from build123d import *

# Parameters (mm, degrees)
SKETCH1_R           = 10
SKETCH1_R_2         = 3.499999985
SKETCH1_R_3         = 3.5
BOSS_EXTRUDE1_DEPTH = 3.175
CUT_EXTRUDE1_DEPTH  = 3.175


with BuildPart() as part:
    # Sketch1 → Boss-Extrude1 (new body)
    # profile 1 of 4: a face of its own
    with BuildSketch(Plane(origin=(0, 79.166310833, -2.766864901), x_dir=(0, -0.03492870325036397, -0.9993898066766781), z_dir=(0, -0.9993898066766781, 0.03492870325036397))):
        with BuildLine():
            ThreePointArc((-118.870418158, 10), (-111.799350346, 7.071067812), (-108.870418158, 0))
            ThreePointArc((-108.870418158, 0), (-111.799350346, -7.071067812), (-118.870418158, -10))
            ThreePointArc((-118.870418158, -10), (4.966133868, -24.680117915), (121.938173717, -67.906722838))
            ThreePointArc((121.938173717, -67.906722838), (119.088657305, -52.269505992), (134.924502551, -53.636363636))
            ThreePointArc((134.924502551, -53.636363636), (119.323202161, 0), (134.924502551, 53.636363636))
            ThreePointArc((134.924502551, 53.636363636), (119.088657305, 52.269505992), (121.938173717, 67.906722838))
            ThreePointArc((121.938173717, 67.906722838), (4.966133868, 24.680117915), (-118.870418158, 10))
        make_face()
    # profile 2 of 4: a face of its own
    with BuildSketch(Plane(origin=(0, 79.166310833, -2.766864901), x_dir=(0, -0.03492870325036397, -0.9993898066766781), z_dir=(0, -0.9993898066766781, 0.03492870325036397))):
        with Locations((-118.870418158, 0)):
            Circle(SKETCH1_R)
        with Locations((-118.870418158, 0)):
            Circle(SKETCH1_R_2, mode=Mode.SUBTRACT)
    # profile 3 of 4: a face of its own
    with BuildSketch(Plane(origin=(0, 79.166310833, -2.766864901), x_dir=(0, -0.03492870325036397, -0.9993898066766781), z_dir=(0, -0.9993898066766781, 0.03492870325036397))):
        with Locations((126.48463259, 59)):
            Circle(SKETCH1_R)
        with Locations((126.48463259, 59)):
            Circle(SKETCH1_R_3, mode=Mode.SUBTRACT)
    # profile 4 of 4: a face of its own
    with BuildSketch(Plane(origin=(0, 79.166310833, -2.766864901), x_dir=(0, -0.03492870325036397, -0.9993898066766781), z_dir=(0, -0.9993898066766781, 0.03492870325036397))):
        with Locations((126.48463259, -59)):
            Circle(SKETCH1_R)
        with Locations((126.48463259, -59)):
            Circle(SKETCH1_R_3, mode=Mode.SUBTRACT)
    extrude(amount=BOSS_EXTRUDE1_DEPTH)

    # Sketch2 → Cut-Extrude1 (cut)
    with BuildSketch(Plane(origin=(0, 75.993248196, -2.655966268), x_dir=(1, 0, 0), z_dir=(0, -0.9993898066766781, 0.034928703250363964))):
        with BuildLine():
            Line((1.5875, 112.870418158), (1.5875, 102.870418158))
            ThreePointArc((1.5875, 102.870418158), (0, 101.282918158), (-1.5875, 102.870418158))
            Line((-1.5875, 102.870418158), (-1.5875, 112.870418158))
            ThreePointArc((-1.5875, 112.870418158), (0, 114.457918158), (1.5875, 112.870418158))
        make_face()
        with BuildLine():
            Line((1.5875, -105.938173717), (1.5875, -115.938173717))
            ThreePointArc((1.5875, -115.938173717), (0, -117.525673717), (-1.5875, -115.938173717))
            Line((-1.5875, -115.938173717), (-1.5875, -105.938173717))
            ThreePointArc((-1.5875, -105.938173717), (0, -104.350673717), (1.5875, -105.938173717))
        make_face()
        with BuildLine():
            Line((1.5875, 58.168270189), (1.5875, 48.168270189))
            ThreePointArc((1.5875, 48.168270189), (0, 46.580770189), (-1.5875, 48.168270189))
            Line((-1.5875, 48.168270189), (-1.5875, 58.168270189))
            ThreePointArc((-1.5875, 58.168270189), (0, 59.755770189), (1.5875, 58.168270189))
        make_face()
        with BuildLine():
            Line((1.5875, 3.46612222), (1.5875, -6.53387778))
            ThreePointArc((1.5875, -6.53387778), (0, -8.12137778), (-1.5875, -6.53387778))
            Line((-1.5875, -6.53387778), (-1.5875, 3.46612222))
            ThreePointArc((-1.5875, 3.46612222), (0, 5.05362222), (1.5875, 3.46612222))
        make_face()
        with BuildLine():
            Line((1.5875, -51.236025749), (1.5875, -61.236025749))
            ThreePointArc((1.5875, -61.236025749), (0, -62.823525749), (-1.5875, -61.236025749))
            Line((-1.5875, -61.236025749), (-1.5875, -51.236025749))
            ThreePointArc((-1.5875, -51.236025749), (0, -49.648525749), (1.5875, -51.236025749))
        make_face()
        with BuildLine():
            Line((38.57145678, -72.525673717), (28.57145678, -72.525673717))
            ThreePointArc((28.57145678, -72.525673717), (26.98395678, -70.938173717), (28.57145678, -69.350673717))
            Line((28.57145678, -69.350673717), (38.57145678, -69.350673717))
            ThreePointArc((38.57145678, -69.350673717), (40.15895678, -70.938173717), (38.57145678, -72.525673717))
        make_face()
        with BuildLine():
            Line((5, -72.525673717), (-5, -72.525673717))
            ThreePointArc((-5, -72.525673717), (-6.5875, -70.938173717), (-5, -69.350673717))
            Line((-5, -69.350673717), (5, -69.350673717))
            ThreePointArc((5, -69.350673717), (6.5875, -70.938173717), (5, -72.525673717))
        make_face()
        with BuildLine():
            Line((-28.57145678, -72.525673717), (-38.57145678, -72.525673717))
            ThreePointArc((-38.57145678, -72.525673717), (-40.15895678, -70.938173717), (-38.57145678, -69.350673717))
            Line((-38.57145678, -69.350673717), (-28.57145678, -69.350673717))
            ThreePointArc((-28.57145678, -69.350673717), (-26.98395678, -70.938173717), (-28.57145678, -72.525673717))
        make_face()
    extrude(amount=-CUT_EXTRUDE1_DEPTH, mode=Mode.SUBTRACT)


solid = part.part
For this review, take the finished solid that the model builds, in its own axes (mm). Give positions to 0.01 mm unless a question says otherwise; leave off trailing zeros. Write each loop counter-clockwise with the first axis right and the second up, starting at its lowest first coordinate (ties: lowest second). Pieces come first, ordered by that corner, then holes. Notation, with made-up numbers: (-14.75, 64) -> (33.25, 64) arc R30 cw to (33.25, 86) -> close; hole circle Ø4 at (55, -21.5). An arc over 180 degrees is marked (long way). Use CSV: the item, a comma, the result in double quotes.
Q1. Take a section at A-A, the plane x = 32. Write out the cut boundary in (y, z).
Conclusion:
outline,"(71.64, -127.16) -> (74.81, -127.27) -> (76.63, -75.25) -> (73.46, -75.14) -> close; (73.57, -71.96) -> (76.74, -72.08) -> (78.04, -34.94) -> (74.87, -34.83) -> close"
Q2. For P1, Ø1, axis at x = -19.5, z = -74.5, coming from the +Y side; P2, Ø3, axis at y = 76.5, z = -4.5, coming from the +X side; P3, Ø1.1, axis at y = 80, z = 48.5, coming from the +X side, all flat-tipped, find the tip position at first contact; note any pin that passes through.
Conclusion:
P1,"y = 76.68"
P2,"x = 24.29"
P3,"x = 14.4"
Q3. Mouldability with a two-part tool opening along Z and no side actions: class faces 1 (the face through (1.05, 81.64, 112.75)), 2 (the face through (60.051, 73.067, -132.456)) as pulls with the +Z half, pulls with the -Z half, needs draft (parallel to the pull), parting line crosses it, or undercut.
Conclusion:
face 1,"undercut"
face 2,"undercut"
Q4. Take a section at B-B, the plane x = -21.5. Write out the cut boundary in (y, z).
Conclusion:
outline,"(71.74, -124.24) -> (74.92, -124.35) -> (79.48, 6.33) -> (76.31, 6.44) -> close"
Q5. To check wall thickness, follow probe 1 along X at (y, z) = (78.75, -5.5); probe 2 along Y at (x, z) = (-23.5, -54); probe 3 along Y at (x, z) = (8, -64.5). State the ranges of each line that lie inside material, in increasing order. Write a range as [from, to].
Conclusion:
probe 1,"[-24.15, -1.59], [1.59, 24.15]"
probe 2,"[74.2, 77.38]"
probe 3,"[73.83, 77.01]"
